Model file for the job. Use its own axes, mm. Give positions to 0.01 mm unless a question says otherwise; leave off trailing zeros. Order: outer loops, then holes, each group sorted by start corner. A loop starts at its lowest first (then second) coordinate and runs counter-clockwise, first axis right, second up. Notation, with made-up numbers: (38, 60) - (85, 60) arc R9 ccw to (85, 71) - close; hole circle Ø5 at (58.25, 40). An arc over 180 degrees is marked (long way). Return JSON: item names as keys, results as strings. Group by question number.
from build123d import *

# Parameters (mm, degrees)
SKETCH_1_W          = 15
SKETCH_1_H          = 4
SKETCH_2_R          = 2.1
CUT_EXTRUDE_1_DEPTH = 10


with BuildPart() as part:
    # 草图1 → 旋转1 (revolve)
    with BuildSketch(Plane.XY, mode=Mode.PRIVATE) as revolve_1_sk:
        with Locations((32.78, 2)):
            Rectangle(SKETCH_1_W, SKETCH_1_H)
    revolve(revolve_1_sk.sketch.rotate(Axis((0, 0, 0), (0, 1, 0)), 90), axis=Axis((0, 0, 0), (0, 1, 0)))

    # 草图2 → 切除-拉伸1 (cut)
    with BuildSketch(Plane(origin=(0, 4, 0), x_dir=(1, 0, 0), z_dir=(0, 1, 0))):
        with Locations(Location((-32.1, 0, 0), (0, 0, 270))):
            Circle(SKETCH_2_R)
        with Locations(Location((-16.05, 27.799415461, 0), (0, 0, 270))):
            Circle(SKETCH_2_R)
        with Locations(Location((16.05, 27.799415461, 0), (0, 0, 270))):
            Circle(SKETCH_2_R)
        with Locations(Location((32.1, 0, 0), (0, 0, 270))):
            Circle(SKETCH_2_R)
        with Locations(Location((16.05, -27.799415461, 0), (0, 0, 270))):
            Circle(SKETCH_2_R)
        with Locations(Location((-16.05, -27.799415461, 0), (0, 0, 270))):
            Circle(SKETCH_2_R)
    extrude(amount=-CUT_EXTRUDE_1_DEPTH, mode=Mode.SUBTRACT)


solid = part.part
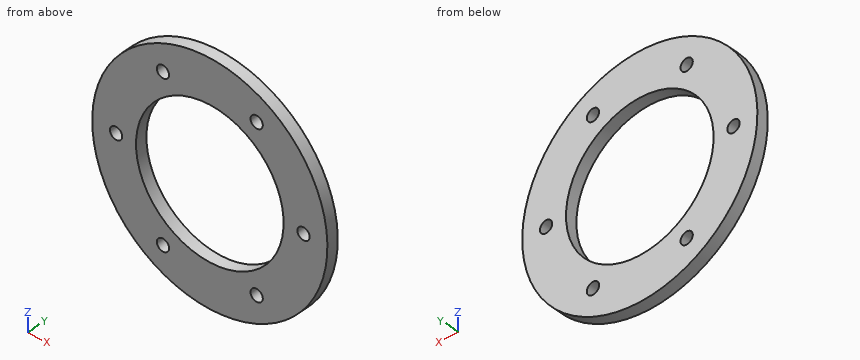
(1) Slice it at D-D (z = -28). Give the cut face in (x, y).
(2) Slice it at B-B (z = 10.5). Give the cut face in (x, y).
(3) Drop a flat-ended pin along its axis: pin 1 Ø3.5 at (x, z) = (-16.05, 27.8) entering from -Y. Give the stop position or say it passes through.
(4) Slice it at A-A (x = 0). Give the cut face in (y, z).
(5) Drill centre lines: L1, parallel to X at y = 1.45, z = 0; L2, parallel to X at y = 0.4, z = -27.5; L3, parallel to Z at x = 15.5, y = 3.45. Where is each one in solid material? Low to high.
(6) Slice it at C-C (y = 2.95). Give the cut face in (x, z).
Result set:
{
 "1": {"outline": "(-28.96, 0) - (-18.14, 0) - (-18.14, 4) - (-28.96, 4) - close; (-13.96, 0) - (13.96, 0) - (13.96, 4) - (-13.96, 4) - close; (18.14, 0) - (28.96, 0) - (28.96, 4) - (18.14, 4) - close"},
 "2": {"outline": "(-38.89, 0) - (-23, 0) - (-23, 4) - (-38.89, 4) - close; (23, 0) - (38.89, 0) - (38.89, 4) - (23, 4) - close"},
 "3": {"pin 1": "passes through"},
 "4": {"outline": "(0, -40.28) - (4, -40.28) - (4, -25.28) - (0, -25.28) - close; (0, 25.28) - (4, 25.28) - (4, 40.28) - (0, 40.28) - close"},
 "5": {"L1": "x = -40.28 to -34.2, -30 to -25.28, 25.28 to 30, 34.2 to 40.28", "L2": "x = -29.43 to -18.13, -13.97 to 13.97, 18.13 to 29.43", "L3": "z = -37.18 to -29.83, -25.77 to -19.97, 19.97 to 25.77, 29.83 to 37.18"},
 "6": {"outline": "circle Ø80.56 at (0, 0); hole circle Ø4.2 at (-32.1, 0); hole circle Ø50.56 at (0, 0); hole circle Ø4.2 at (-16.05, -27.8); hole circle Ø4.2 at (-16.05, 27.8); hole circle Ø4.2 at (16.05, -27.8); hole circle Ø4.2 at (16.05, 27.8); hole circle Ø4.2 at (32.1, 0)"}
}
